from build123d import *

# Parameters (mm, degrees)
SKETCH1_R                = 7.9375
SKETCH1_R_2              = 3.175
BOSS_EXTRUDE1_DEPTH      = 3.175
BOSS_EXTRUDE2_DEPTH      = 3.175
BOSS_EXTRUDE2_DEPTH_BACK = 6.35
SKETCH2_R                = 4.7625
SKETCH2_R_2              = 3.175


with BuildPart() as part:
    # Sketch1 → Boss-Extrude1 (new body)
    with BuildSketch(Plane(origin=(0, 0, 0), x_dir=(1, 0, 0), z_dir=(0, 1, 0))):
        with Locations(Location((0, 0, 0), (0, 0, 270))):
            Circle(SKETCH1_R)
        with Locations(Location((0, 0, 0), (0, 0, 270))):
            Circle(SKETCH1_R_2, mode=Mode.SUBTRACT)
    extrude(amount=BOSS_EXTRUDE1_DEPTH)

    # Sketch2 → Boss-Extrude2 (add, two sides: drawn at the far end of the back side and taken through both)
    with BuildSketch(Plane(origin=(0, 3.175, 0), x_dir=(1, 0, 0), z_dir=(0, 1, 0)).offset(-BOSS_EXTRUDE2_DEPTH_BACK)):
        with Locations(Location((0, 0, 0), (0, 0, 270))):
            Circle(SKETCH2_R)
        with Locations(Location((0, 0, 0), (0, 0, 270))):
            Circle(SKETCH2_R_2, mode=Mode.SUBTRACT)
    extrude(amount=BOSS_EXTRUDE2_DEPTH + BOSS_EXTRUDE2_DEPTH_BACK)


solid = part.part
Source: CAD feature listing. Evaluate the final solid. Frame: model axes, mm. A direction names the side the tool comes from. Give positions to 0.01 mm unless a question says otherwise; leave off trailing zeros. Answer as a JSON object with one key per item and string values.
Q1. Mould query, pull axis Z, two halves, no side actions, for faces 3 (the face through (-5, 0, 0)), 4 (the face through (-1.93, 1.52, -2.52)), 5 (the face through (-7.75, 1.57, -1.72)). Classes: +Z half, -Z half, draft (parallel to the pull), parting line (faces both ways), or undercut.
Geometry check:
{"face 3": "draft", "face 4": "undercut", "face 5": "parting line"}
Q2. Ray query, line 1 along X through (y, z) = (-0.5, 0) (1 decimal); line 2 along X through (y, z) = (0.5, 0) (1 decimal); line 3 along Y through (x, z) = (-5.25, -0.75) (3 decimals). Return the intervals inside material, ascending.
Geometry check:
{"line 1": "x = -4.8 to -3.2, 3.2 to 4.8", "line 2": "x = -7.9 to -3.2, 3.2 to 7.9", "line 3": "y = 0 to 3.175"}
Q3. Contact query for flat-ended pins moving along their axis: P1, Ø2, axis at x = 5, y = 3, coming from the +Z side; P2, Ø3, axis at y = 3, z = 6, coming from the +X side; P3, Ø1, axis at x = -2, z = 6, coming from the +Y side (3 decimals). Output: stop coordinate, or through.
Geometry check:
{"P1": "stops at z = 6.86", "P2": "stops at x = 6.54", "P3": "stops at y = 3.175"}
Q4. Access query for faces 1 (the face through (-2.9, 4.74, -3.78)), 2 (the face through (-2.9, -1.61, -3.78)). Directions: +Z, -Z, +X, -X, +Y, -Y. A direction counts if a zero-diameter tool reaches every point of the face in a straight line with its end or side. Return the directions, or none.
Geometry check:
{"face 1": "+Y", "face 2": "-Y"}
